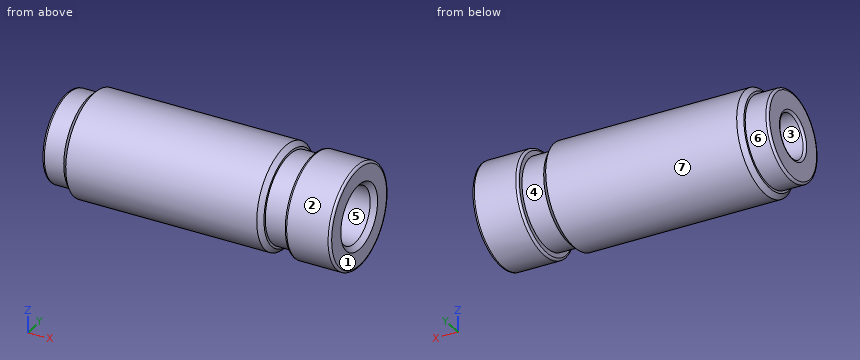
```python
from build123d import *

# Parameters (mm, degrees)
FURO_ROSCADO_DE_M14X2_01_D           = 12
FURO_ROSCADO_DE_M14X2_01_DEPTH       = 53.5
FURO_ROSCADO_DE_M14X2_01_CSINK_D     = 14.05
FURO_ROSCADO_DE_M14X2_01_CSINK_ANGLE = 90
FURO_ROSCADO_DE_M14X2_01_TIP         = 3.605163714
FURO1_D                              = 9.4
FURO1_DEPTH                          = 10
CHANFRO1_SIZE                        = 1
FILETE1_R                            = 0.5


with BuildPart() as part:
    # Esboço1 → Revolução1 (revolve)
    with BuildSketch(Plane.XY, mode=Mode.PRIVATE) as revolu_o1_sk:
        Polygon((0, 0), (63.5, 0), (63.5, 11), (53.5, 11), (53.5, 9.5), (48.5, 9.5), (48.5, 11), (5, 11), (5, 9.5), (0, 9.5), align=None)
    revolve(revolu_o1_sk.sketch.rotate(Axis((0, 0, 0), (1, 0, 0)), 90), axis=Axis((0, 0, 0), (1, 0, 0)))

    # Furo roscado de M14x2.01
    with Locations(Plane(origin=(63.5, 0, 0), x_dir=(0, 0, -1), z_dir=(1, 0, 0))):
        with Locations((0, 0)):
            CounterSinkHole(FURO_ROSCADO_DE_M14X2_01_D / 2, FURO_ROSCADO_DE_M14X2_01_CSINK_D / 2, depth=FURO_ROSCADO_DE_M14X2_01_DEPTH, counter_sink_angle=FURO_ROSCADO_DE_M14X2_01_CSINK_ANGLE)
            with Locations((0, 0, -(FURO_ROSCADO_DE_M14X2_01_DEPTH + FURO_ROSCADO_DE_M14X2_01_TIP / 2))):  # 118° drill point
                Cone(0, FURO_ROSCADO_DE_M14X2_01_D / 2, FURO_ROSCADO_DE_M14X2_01_TIP, mode=Mode.SUBTRACT)

    # Furo1
    with Locations(Plane.ZY):
        with Locations((0, 0)):
            Hole(FURO1_D / 2, depth=FURO1_DEPTH)

    # Chanfro1
    chanfro1_edges = [part.edges().sort_by_distance(p)[0] for p in [
        (5, 0, -11),
        (48.5, 0, -11),
    ]]
    chamfer(chanfro1_edges, length=CHANFRO1_SIZE)

    # Filete1
    filete1_edges = [part.edges().sort_by_distance(p)[0] for p in [
        (63.5, 0, -11),
        (0, 0, 4.7),
        (0, 0, -9.5),
        (53.5, 0, -11),
    ]]
    fillet(filete1_edges, radius=FILETE1_R)


solid = part.part
```
Model file for the job. Use its own axes, mm. Face numbers are marked on the shaded views. A direction names the side the tool comes from. Give positions to 0.01 mm unless a question says otherwise; leave off trailing zeros. Write each loop counter-clockwise with the first axis right and the second up, starting at its lowest first coordinate (ties: lowest second). Pieces come first, ordered by that corner, then holes. Notation, with made-up numbers: M 87,-9 L 94,-9 A12 cw 94,2 Z; hole C -21,32 d10. An arc over 180 degrees is marked long. Use a Markdown table: item, result.
1) Cut at A-A (x = 46.5). List the corners of the cut face in (y, z), and give its area (3 significant figures).
Responses:
| item | result |
|---|---|
| outline | C 0,0 d22; hole C 0,0 d12 |
| area | 267 mm2 |
2) Pin check, flat tips, straight feed: pin 1 (1 mm diameter, centred on y = -6.5, z = 0, fed in from +X) (3 decimals); pin 2 (1.5 mm diameter, centred on x = 29.5, y = -4.5, fed in from -Z); pin 3 (10 mm diameter, centred on x = 45.5, z = 6, fed in from -Y). Stop position of each tip, or through.
Responses:
| item | result |
|---|---|
| pin 1 | stops at x = 63.475 |
| pin 2 | stops at z = -10.34 |
| pin 3 | stops at y = -10.95 |
3) Drill centre lines: line 1 (Y direction, x = 2.5, z = 0); line 2 (Y direction, x = 35, z = 0); line 3 (X direction, y = 8.5, z = 5.25). Where is each one in solid material? Low to high. Write a range as from..to.
Responses:
| item | result |
|---|---|
| line 1 | y = -9.5..-4.7, 4.7..9.5 |
| line 2 | y = -11..-6, 6..11 |
| line 3 | x = 5..48.5, 53.5..63.5 |
4) Cut at B-B (x = 7.5). List the corners of the cut face in (y, z).
Responses:
| item | result |
|---|---|
| outline | C 0,0 d22; hole C 0,0 d9.4 |
5) Pull direction Z, two halves, no side cores. Call the marked faces 1, 2 and 3: +Z half, -Z half, draft (parallel to the pull), parting line (faces both ways), or undercut.
Responses:
| item | result |
|---|---|
| face 1 | draft |
| face 2 | parting line |
| face 3 | undercut |
6) Tool access for the marked faces 4, 5, 6 and 7: list every direction of +Z, -Z, +X, -X, +Y, -Y with a clear straight run to the whole face (end or side of a thin tool).
Responses:
| item | result |
|---|---|
| face 4 | none |
| face 5 | +X |
| face 6 | -X |
| face 7 | +X, -X |
